Build history of the part. All positions in model axes, mm. A direction names the side the tool comes from. Round coordinates to 2 decimals unless told otherwise and drop trailing zeros. Write each loop counter-clockwise with the first axis right and the second up, starting at its lowest first coordinate (ties: lowest second). Pieces come first, ordered by that corner, then holes. Notation, with made-up numbers: (72.25, 57.5) - (93.25, 57.5) arc R4 cw to (93.25, 62.5) - close; hole circle Ø4 at (-17, 13.25). An arc over 180 degrees is marked (long way). Answer as a JSON object with one key per item and string values. Group by question number.
Item 1: Probe line 1 (Y direction, x = 4, z = 1.3); line 2 (Y direction, x = 14, z = 2.2); line 3 (X direction, y = 8.25, z = 1.35). List the from-to ranges inside material, lowest first. Write a range as from..to.
Item 2: Slice it at D-D, the plane x = 12.75. List the corners of the cut face in (y, z), then the cut area to 3 significant figures.
Item 3: Slice it at A-A, the plane y = 14. List the corners of the cut face in (x, z), then the cut area to 3 significant figures.
Item 4: Slice it at B-B, the plane x = 4. List the corners of the cut face in (y, z), then the cut area to 3 significant figures.
Item 5: Slice it at C-C, the plane z = 4.3. List the corners of the cut face in (x, y).
Item 6: Two-plate mould, pull along X, no slides. Class faces 4 (the flat face through (10, 9, 0)), 5 (the flat face through (14, 15.65, 4)), 6 (the flat face through (8, 9, 4)), 7 (the flat face through (16, 9, 2)): +X half, -X half, draft (parallel to the pull), parting line (faces both ways), or undercut.
Item 7: Flat gauge pins, fed straight in: pin 1 (0.8 mm diameter, centred on x = 16.5, y = 11.5, fed in from +Z); pin 2 (1 mm diameter, centred on y = 7.5, z = 3.5, fed in from -X). Where does each tip first touch, or does it go through?
Item 8: Which spindle directions (+Z, -Z, +X, -X, +Y, -Y) get a long thin tool onto all of the face, cutting with end or side? Do faces 1 (the flat face through (10.85, 9, 4)), 2 (the flat face through (15.5, 9, 1)), 3 (the flat face through (4, 9, 2)). Say none if no direction does.
Autodesk Inventor part; units mm, degrees
ref_plane "YZ Plane" through (0, 0, 0) normal (1, 0, 0) x (0, 1, 0)
ref_plane "XZ Plane" through (0, 0, 0) normal (0, 1, 0) x (-1, 0, 0)
ref_plane "XY Plane" through (0, 0, 0) normal (0, 0, 1) x (1, 0, 0)
sketch "Sketch1" plane through (0, 0, 0) normal (0, 0, 1) x (1, 0, 0)
  line L0 (0, 0) -> (20, 0)
  line L1 (20, 0) -> (20, 18)
  line L2 (20, 18) -> (0, 18)
  line L3 (0, 18) -> (0, 0)
  line L4 (12.5, 2.35) -> (15.5, 2.35)
  line L5 (15.5, 2.35) -> (15.5, 15.65)
  line L6 (15.5, 15.65) -> (12.5, 15.65)
  line L7 (12.5, 15.65) -> (12.5, 2.35)
  circle A0 centre (4, 14) radius 1.7
  circle A1 centre (4, 4) radius 1.7
  line L8 (20, 18) -> (8, 18)
  line L9 (8, 18) -> (8, 0)
  line L10 (8, 0) -> (20, 0)
  line L11 (20, 0) -> (20, 18)
  line L12 (10.85, 15.65) -> (17.15, 15.65)
  line L13 (17.15, 15.65) -> (17.15, 2.35)
  line L14 (17.15, 2.35) -> (10.85, 2.35)
  line L15 (10.85, 2.35) -> (10.85, 15.65)
  point P0 (15.5, 9)
  point P1 (20, 9)
  point P2 (14, 15.65)
  point P3 (14, 18)
  point P4 (17.15, 9)
  point P5 (20, 9)
  point P6 (14, 15.65)
  dimension "d0" = 20
  dimension "d1" = 18
  dimension "d3" = 3
  dimension "d5" = 3.4
  dimension "d6" = 3.4
  dimension "d7" = 4
  dimension "d8" = 4
  dimension "d9" = 10
  dimension "d20" = 12
  dimension "d21" = 6.3
  dimension "d22" = 13.3
extrude "Extrusion1" add sketch "Sketch1" along normal blind 2 contours L3 L2 L9 L0 | L9 L2 L1 L0 | L14 L15 L12 L7 | L5 L12 L13 L14
extrude "Extrusion3" add sketch "Sketch1" along normal blind 6 contours L9 L2 L1 L0
properties part number "switch lever 2"
Geometry says:
{
 "1": {"line 1": "y = 0..2.3, 5.7..12.3, 15.7..18", "line 2": "y = 0..2.35, 15.65..18", "line 3": "x = 0..12.5, 15.5..20"},
 "2": {"outline": "(0, 0) - (2.35, 0) - (2.35, 6) - (0, 6) - close; (15.65, 0) - (18, 0) - (18, 6) - (15.65, 6) - close", "area": "28.2 mm^2"},
 "3": {"outline": "(0, 0) - (2.3, 0) - (2.3, 2) - (0, 2) - close; (5.7, 0) - (12.5, 0) - (12.5, 2) - (10.85, 2) - (10.85, 6) - (8, 6) - (8, 2) - (5.7, 2) - close; (15.5, 0) - (20, 0) - (20, 6) - (17.15, 6) - (17.15, 2) - (15.5, 2) - close", "area": "50.0 mm^2"},
 "4": {"outline": "(0, 0) - (2.3, 0) - (2.3, 2) - (0, 2) - close; (5.7, 0) - (12.3, 0) - (12.3, 2) - (5.7, 2) - close; (15.7, 0) - (18, 0) - (18, 2) - (15.7, 2) - close", "area": "22.4 mm^2"},
 "5": {"outline": "(8, 0) - (20, 0) - (20, 18) - (8, 18) - close; hole (10.85, 2.35) - (17.15, 2.35) - (17.15, 15.65) - (10.85, 15.65) - close"},
 "6": {"face 4": "draft", "face 5": "undercut", "face 6": "-X half", "face 7": "undercut"},
 "7": {"pin 1": "stops at z = 2", "pin 2": "stops at x = 8"},
 "8": {"face 1": "+Z", "face 2": "+Z, -Z", "face 3": "+Z, -X, +Y, -Y"}
}
